CAD build for the part. Positions are in the model's coordinates, mm. Face numbers are marked on the shaded views. A direction names the side the tool comes from. Round coordinates to 2 decimals unless told otherwise and drop trailing zeros. Write each loop counter-clockwise with the first axis right and the second up, starting at its lowest first coordinate (ties: lowest second). Pieces come first, ordered by that corner, then holes. Notation, with made-up numbers: (-37, 70) - (-10, 70) arc R29 cw to (-10, 104) - close; hole circle Ø11 at (65, 75.5). An arc over 180 degrees is marked (long way). Answer in a Markdown table with one row per item.
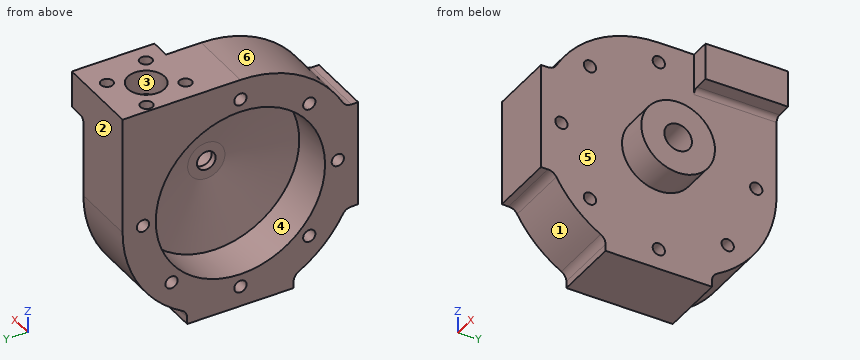
```python
from build123d import *

# Parameters (mm, degrees)
HOUSING_2_DEPTH          = 44.45
SKETCH2_R                = 43.815
IMPELLER_CUT_DEPTH       = 22.4028
SKETCH4_R                = 4.826
INLET_CUT_DEPTH          = 19.8628
SKETCH6_R                = 3.175
FASTENER_BORE_DEPTH      = 116.84
FASTENER_PATTERN_COUNT   = 8
SKETCH7_R                = 100.114274451
SKETCH7_R_2              = 19.05
MASS_REDUCTION_CUT_DEPTH = 10.414
SKETCH11_R               = 19.05
SKETCH11_R_2             = 4.826
BOSS_EXTRUDE1_DEPTH      = 6.35
SKETCH14_R               = 2.38125
CUT_EXTRUDE3_DEPTH       = 99.06
SKETCH15_R               = 9.525
CUT_EXTRUDE4_DEPTH       = 25.4
BOSS_EXTRUDE2_START      = 12.7
SKETCH16_R               = 9.525
SKETCH16_R_2             = 6.35
BOSS_EXTRUDE2_DEPTH      = 12.7
SKETCH18_W               = 10.060456949
SKETCH18_H               = 42.763815868
BOSS_EXTRUDE3_DEPTH      = 19.05
FILLET7_R                = 2.54
SKETCH19_R               = 3.175
CUT_EXTRUDE5_DEPTH       = 15.24
FILLET9_R                = 5.08
SKETCH22_R               = 7.1374
CUT_EXTRUDE8_DEPTH       = 17.78
CIRPATTERN2_COUNT        = 4


with BuildPart() as part:
    # Sketch1 → Housing 2 (new body)
    with BuildSketch(Plane(origin=(0, 0, 0), x_dir=(0, 0, -1), z_dir=(1, 0, 0))):
        with BuildLine():
            Line((-60.96, 0), (-60.96, 60.96))
            Line((-60.96, 60.96), (0, 60.96))
            ThreePointArc((0, 60.96), (31.907091375, 51.942844743), (54.374839025, 27.559))
            Line((54.374839025, 27.559), (60.96, 27.559))
            Line((60.96, 27.559), (60.96, -27.559))
            Line((60.96, -27.559), (54.374839025, -27.559))
            ThreePointArc((54.374839025, -27.559), (43.093739421, -43.116716279), (27.530012063, -54.389521379))
            Line((27.530012063, -54.389521379), (27.530012063, -60.96))
            Line((27.530012063, -60.96), (-27.530012063, -60.96))
            Line((-27.530012063, -60.96), (-27.530012063, -54.389521379))
            ThreePointArc((-27.530012063, -54.389521379), (-51.934339003, -31.920934077), (-60.96, 0))
        make_face()
    extrude(amount=HOUSING_2_DEPTH)

    # Sketch2 → Impeller Cut (cut)
    with BuildSketch(Plane.ZY):
        Circle(SKETCH2_R)
    extrude(amount=-IMPELLER_CUT_DEPTH, mode=Mode.SUBTRACT)

    # Sketch3 → Impeller Angle Cut (revolve, cut)
    with BuildSketch(Plane.XY, mode=Mode.PRIVATE) as impeller_angle_cut_sk:
        Polygon((29.602825054, 9.641475923), (22.4028, 43.815), (22.225, 0), (29.602825054, 0), align=None)
    revolve(impeller_angle_cut_sk.sketch.rotate(Axis((22.225, 0, 0), (1, 0, 0)), 180), axis=Axis((22.225, 0, 0), (1, 0, 0)), mode=Mode.SUBTRACT)

    # Sketch4 → Inlet Cut (cut)
    with BuildSketch(Plane.ZY.offset(-29.602825054)):
        Circle(SKETCH4_R)
    extrude(amount=-INLET_CUT_DEPTH, mode=Mode.SUBTRACT)

    # Sketch6 → Fastener Bore (cut)
    with BuildSketch(Plane(origin=(44.45, 0, 0), x_dir=(0, 0, -1), z_dir=(1, 0, 0))):
        with Locations((50.419, 0)):
            Circle(SKETCH6_R)
    fastener_bore = extrude(amount=-FASTENER_BORE_DEPTH, mode=Mode.SUBTRACT)

    # Fastener Pattern: Fastener Bore ×8 about axis, 1 skipped
    fastener_pattern_axis = Axis((0, 0, 0), (-1, 0, 0))
    add([fastener_bore.rotate(fastener_pattern_axis, i * 360 / FASTENER_PATTERN_COUNT) for i in range(1, FASTENER_PATTERN_COUNT) if i not in (5,)], mode=Mode.SUBTRACT)

    # Sketch7 → Mass Reduction Cut (cut)
    with BuildSketch(Plane(origin=(44.45, 0, 0), x_dir=(0, 0, -1), z_dir=(1, 0, 0))):
        Circle(SKETCH7_R)
        Circle(SKETCH7_R_2, mode=Mode.SUBTRACT)
    extrude(amount=-MASS_REDUCTION_CUT_DEPTH, mode=Mode.SUBTRACT)

    # Sketch11 → Boss-Extrude1 (add)
    with BuildSketch(Plane(origin=(44.45, 0, 0), x_dir=(0, 0, -1), z_dir=(1, 0, 0))):
        Circle(SKETCH11_R)
        with Locations(Location((0, 0, 0), (0, 0, 180))):
            Circle(SKETCH11_R_2, mode=Mode.SUBTRACT)
    extrude(amount=BOSS_EXTRUDE1_DEPTH)

    # Sketch14 → Cut-Extrude3 (cut)
    with BuildSketch(Plane.XY):
        with Locations(Location((19.558, 37.084, 0), (0, 0, 180))):
            Circle(SKETCH14_R)
    extrude(amount=CUT_EXTRUDE3_DEPTH, mode=Mode.SUBTRACT)

    # Sketch15 → Cut-Extrude4 (cut)
    with BuildSketch(Plane.XY.offset(60.96)):
        with Locations((19.558, 37.084)):
            Circle(SKETCH15_R)
    extrude(amount=-CUT_EXTRUDE4_DEPTH, mode=Mode.SUBTRACT)

    # Sketch16 → Boss-Extrude2 (add)
    with BuildSketch(Plane.XY.offset(35.56).offset(BOSS_EXTRUDE2_START)):
        with Locations((19.558, 37.084)):
            Circle(SKETCH16_R)
        with Locations(Location((19.558, 37.084, 0), (0, 0, 180))):
            Circle(SKETCH16_R_2, mode=Mode.SUBTRACT)
    extrude(amount=-BOSS_EXTRUDE2_DEPTH)

    # Sketch18 → Boss-Extrude3 (add)
    with BuildSketch(Plane.XY.offset(60.96)):
        with Locations((39.066228475, 39.578092066)):
            Rectangle(SKETCH18_W, SKETCH18_H)
    extrude(amount=-BOSS_EXTRUDE3_DEPTH)

    # Fillet7
    fillet7_edges = [part.edges().sort_by_distance(p)[0] for p in [
        (34.036, 39.578092066, 41.91),
    ]]
    fillet(fillet7_edges, radius=FILLET7_R)

    # Sketch19 → Cut-Extrude5 (cut)
    with BuildSketch(Plane.XY.offset(60.96)):
        with Locations((34.640612035, 28.263568969)):
            Circle(SKETCH19_R)
    cut_extrude5 = extrude(amount=-CUT_EXTRUDE5_DEPTH, mode=Mode.SUBTRACT)

    # Fillet9
    fillet9_edges = [part.edges().sort_by_distance(p)[0] for p in [
        (17.018, 27.559, -54.374839025),
        (17.018, -27.559, -54.374839025),
        (17.018, -54.389521379, -27.530012063),
        (17.018, -54.389521379, 27.530012063),
    ]]
    fillet(fillet9_edges, radius=FILLET9_R)

    # Sketch22 → Cut-Extrude8 (cut)
    with BuildSketch(Plane(origin=(50.8, 0, 0), x_dir=(0, 0, -1), z_dir=(1, 0, 0))):
        Circle(SKETCH22_R)
    extrude(amount=-CUT_EXTRUDE8_DEPTH, mode=Mode.SUBTRACT)

    # CirPattern2: Cut-Extrude5 ×4 about axis
    cirpattern2_axis = Axis((19.558, 37.084, 0), (0, 0, 1))
    for i in range(1, CIRPATTERN2_COUNT):
        add(cut_extrude5.rotate(cirpattern2_axis, i * 360 / CIRPATTERN2_COUNT), mode=Mode.SUBTRACT)


solid = part.part
```
Q1. 3-axis set-ups, long thin cutter, end or side, ignore diameter. For the marked faces 4, 5 and 6: which of +Z, -Z, +X, -X, +Y, -Y reach the whole face in a straight line?
Computed:
| item | result |
|---|---|
| face 4 | -X |
| face 5 | +X |
| face 6 | +Z, +X, -X, -Y |
Q2. Flat gauge pins, fed straight in: pin 1 (4 mm diameter, centred on y = 35.65, z = -35.65, fed in from +X); pin 2 (1 mm diameter, centred on y = -40, z = 8.5, fed in from +X); pin 3 (8 mm diameter, centred on y = -24.5, z = 26.5, fed in from -X); pin 4 (1.8 mm diameter, centred on x = 13, y = -58.5, fed in from +Z). Where does each tip first touch, or does it go through?
Computed:
| item | result |
|---|---|
| pin 1 | passes through |
| pin 2 | stops at x = 34.04 |
| pin 3 | stops at x = 23.19 |
| pin 4 | stops at z = 27.53 |
Q3. Saw through at A-A on y = 52. List the corners of the cut face in (x, z).
Computed:
| item | result |
|---|---|
| outline | (0, -31.81) - (34.04, -31.81) - (34.04, -2.75) - (0, -2.75) - close; (0, 2.75) - (34.04, 2.75) - (34.04, 39.37) arc R2.54 cw to (36.58, 41.91) - (44.1, 41.91) - (44.1, 60.96) - (31.55, 60.96) - (31.55, 45.72) - (25.21, 45.72) - (25.21, 60.96) - (0, 60.96) - close |
Q4. Pull direction Y, two halves, no side cores. Call the marked faces 1, 2 and 3: released by +Y, released by -Y, zero draft, split by the parting line, or undercut.
Computed:
| item | result |
|---|---|
| face 1 | released by -Y |
| face 2 | released by +Y |
| face 3 | undercut |
Q5. Saw through at B-B on z = -49.5. List the corners of the cut face in (x, y), then the cut area to 3 significant figures.
Computed:
| item | result |
|---|---|
| outline | (0, -35.58) - (34.04, -35.58) - (34.04, -3.04) - (0, -3.04) - close; (0, 3.04) - (34.04, 3.04) - (34.04, 35.58) - (0, 35.58) - close |
| area | 2,220 mm2 |
Q6. Drill centre lines: line 1 (Z direction, x = 10, y = 37); line 2 (Z direction, x = 15.5, y = -38.5); line 3 (Y direction, x = 9.5, z = 51.5). Where is each one in solid material? Low to high.
Computed:
| item | result |
|---|---|
| line 1 | z = -48.45 to -38.53, -32.78 to -23.47, 23.47 to 60.96 |
| line 2 | z = -47.26 to -37.05, -34.25 to -20.92, 20.92 to 34.25, 37.05 to 47.26 |
| line 3 | y = -32.62 to -2.99, 2.99 to 19.08, 24.93 to 60.96 |
